Geometry: final body of the model. Coordinates: model frame, mm. Face numbers are marked on the shaded views. A direction names the side the tool comes from. Give positions to 0.01 mm unless a question says otherwise; leave off trailing zeros. Write each loop counter-clockwise with the first axis right and the second up, starting at its lowest first coordinate (ties: lowest second). Pieces come first, ordered by that corner, then holes. Notation, with made-up numbers: (77.5, 82) - (81.5, 82) arc R32 ccw to (81.5, 115) - close; hole circle Ø4 at (51, 8). An arc over 180 degrees is marked (long way). Use CSV: the item, a comma, the result in double quotes. Start each with the question number.
(1) First-contact query: pin 1 Ø4.5 at (x, z) = (46.26, -48.97) entering from -Y; pin 2 Ø6 at (x, z) = (-56, 71) entering from -Y; pin 3 Ø4 at (x, z) = (-88.5, 41) entering from +Y. Flat tips, straight axial feed; report the tip coordinate or a pass-through.
(2) Section C-C on z = 53.5. Output: boundary loops of the cut face in (x, y), and give its area (3 significant figures).
(3) Section A-A on x = 2.54. Output: boundary loops of the cut face in (y, z), and give its area (3 significant figures).
(4) Reachability of the marked faces 3 and 4 from +Z, -Z, +X, -X, +Y, -Y: full face, straight path, thin tool, end or side. Return the list, or none.
(5) Section B-B on y = 17.75. Count the separate pieces of the cut face and the enclosed holes in it, and give its area (3 significant figures).
(6) Draft query along X for the marked faces 1 and 2. Return one class per face: released by +X, released by -X, zero draft, split by the parting line, or undercut.
(7) Section D-D on x = -19. Output: boundary loops of the cut face in (y, z).
(8) Line query: probe 1 along Z at (x, y) = (-123.5, 1.25); probe 2 along Z at (x, y) = (40.64, 4.5); probe 3 along Y at (x, z) = (36, 3.5). Output: solid intervals per line, ascending. Write a range as [from, to].
from build123d import *

# Parameters (mm, degrees)
SKETCH2_W           = 194.056
SKETCH2_H           = 152.4
BOSS_EXTRUDE1_DEPTH = 6.35
SKETCH3_R           = 3.175
CUT_EXTRUDE1_DEPTH  = 6.35
SKETCH4_W           = 24.892
SKETCH4_H           = 13.97
SKETCH4_W_2         = 25
BOSS_EXTRUDE2_DEPTH = 19.05
SKETCH5_R           = 2.5
CUT_EXTRUDE2_DEPTH  = 26.4


with BuildPart() as part:
    # Sketch2 → Boss-Extrude1 (new body)
    with BuildSketch(Plane(origin=(0, 0, 0), x_dir=(1, 0, 0), z_dir=(0, 1, 0))):
        with Locations((-43.688, -19.614444444)):
            Rectangle(SKETCH2_W, SKETCH2_H)
    extrude(amount=BOSS_EXTRUDE1_DEPTH)

    # Sketch3 → Cut-Extrude1 (cut)
    with BuildSketch(Plane(origin=(0, 6.35, 0), x_dir=(1, 0, 0), z_dir=(0, 1, 0))):
        with Locations((2.54, -70.414444444)):
            Circle(SKETCH3_R)
        with Locations((2.54, 31.185555556)):
            Circle(SKETCH3_R)
        with Locations((40.64, 31.185555556)):
            Circle(SKETCH3_R)
        with Locations((40.64, -70.414444444)):
            Circle(SKETCH3_R)
    extrude(amount=-CUT_EXTRUDE1_DEPTH, mode=Mode.SUBTRACT)

    # Sketch4 → Boss-Extrude2 (add)
    with BuildSketch(Plane(origin=(0, 6.35, 0), x_dir=(1, 0, 0), z_dir=(0, 1, 0))):
        with Locations((40.894, -88.829444444)):
            Rectangle(SKETCH4_W, SKETCH4_H)
        with Locations((-128.216, -88.829444444)):
            Rectangle(SKETCH4_W_2, SKETCH4_H)
        with Locations((-128.216, 49.600555556)):
            Rectangle(SKETCH4_W_2, SKETCH4_H)
        with Locations((40.894, 49.600555556)):
            Rectangle(SKETCH4_W, SKETCH4_H)
    extrude(amount=BOSS_EXTRUDE2_DEPTH)

    # Sketch5 → Cut-Extrude2 (cut, through all)
    with BuildSketch(Plane(origin=(0, 25.4, 0), x_dir=(1, 0, 0), z_dir=(0, 1, 0))):
        with Locations((-133.526, -88.194444444)):
            Circle(SKETCH5_R)
        with Locations((-123.526, -88.194444444)):
            Circle(SKETCH5_R)
        with Locations((-133.526, 48.965555556)):
            Circle(SKETCH5_R)
        with Locations((-123.526, 48.965555556)):
            Circle(SKETCH5_R)
        with Locations((36.258, 48.965555556)):
            Circle(SKETCH5_R)
        with Locations((46.258, 48.965555556)):
            Circle(SKETCH5_R)
        with Locations((36.258, -88.194444444)):
            Circle(SKETCH5_R)
        with Locations((46.258, -88.194444444)):
            Circle(SKETCH5_R)
    extrude(amount=-CUT_EXTRUDE2_DEPTH, mode=Mode.SUBTRACT)


solid = part.part
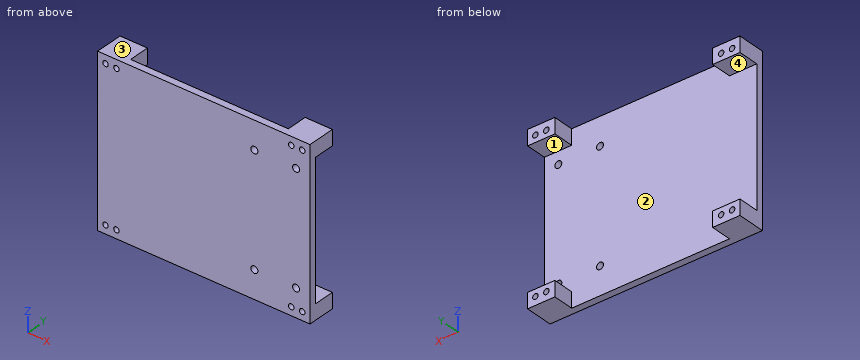
Check values:
1,pin 1,"passes through"
1,pin 2,"stops at y = 0"
1,pin 3,"stops at y = 6.35"
2,outline,"(-140.72, 0) - (53.34, 0) - (53.34, 6.35) - (-140.72, 6.35) - close"
2,area,"1,230 mm²"
3,outline,"(0, -56.59) - (6.35, -56.59) - (6.35, -34.36) - (0, -34.36) - close; (0, -28.01) - (6.35, -28.01) - (6.35, 67.24) - (0, 67.24) - close; (0, 73.59) - (6.35, 73.59) - (6.35, 95.81) - (0, 95.81) - close"
3,area,"887 mm²"
4,face 3,"+Z, +X, -X, +Y, -Y"
4,face 4,"+X, -X, +Y"
5,separate pieces,"4"
5,enclosed holes,"8"
5,area,"1,240 mm²"
6,face 1,"zero draft"
6,face 2,"undercut"
7,outline,"(0, -56.59) - (6.35, -56.59) - (6.35, 95.81) - (0, 95.81) - close"
8,probe 1,"z = [-56.59, -51.47], [-46.47, 85.69], [90.69, 95.81]"
8,probe 2,"z = [-56.59, -34.36], [-28.01, 67.24], [73.59, 95.81]"
8,probe 3,"y = [0, 6.35]"
